Here's how the part is built. I have some questions about the finished solid (model axes, mm). A direction names the side the tool comes from. Give positions to 0.01 mm unless a question says otherwise; leave off trailing zeros. Order: outer loops, then holes, each group sorted by start corner. A loop starts at its lowest first (then second) coordinate and runs counter-clockwise, first axis right, second up.
from build123d import *

# Parameters (mm, degrees)
SKETCH1_R           = 3
SKETCH1_R_2         = 1.2
SKETCH1_R_3         = 6.35
SKETCH1_W           = 5
SKETCH1_H           = 15
SKETCH1_W_2         = 10
SKETCH1_H_2         = 17.5
BOSS_EXTRUDE1_DEPTH = 5
SKETCH2_W           = 38
SKETCH2_H           = 55
BOSS_EXTRUDE2_DEPTH = 5
FILLET1_R           = 5


with BuildPart() as part:
    # Sketch1 → Boss-Extrude1 (new body)
    with BuildSketch(Plane.XY):
        Polygon((-23.5, 65), (23.5, 65), (23.5, 0), (0, 0), (-23.5, 0), align=None)
        with Locations((16, 51)):
            Circle(SKETCH1_R, mode=Mode.SUBTRACT)
        with Locations((16, 19.2)):
            Circle(SKETCH1_R_2, mode=Mode.SUBTRACT)
        with Locations((16, 59)):
            Circle(SKETCH1_R_2, mode=Mode.SUBTRACT)
        with Locations(Location((-16, 59, 0), (0, 0, 180))):
            Circle(SKETCH1_R_2, mode=Mode.SUBTRACT)
        with Locations(Location((-16, 19.2, 0), (0, 0, 180))):
            Circle(SKETCH1_R_2, mode=Mode.SUBTRACT)
        with Locations(Location((-16, 51, 0), (0, 0, 180))):
            Circle(SKETCH1_R, mode=Mode.SUBTRACT)
        with Locations((0, 15)):
            Circle(SKETCH1_R_3, mode=Mode.SUBTRACT)
        with Locations((16, 33.5)):
            Rectangle(SKETCH1_W, SKETCH1_H, mode=Mode.SUBTRACT)
        with Locations((-2.5, 45.25)):
            Rectangle(SKETCH1_W_2, SKETCH1_H_2, mode=Mode.SUBTRACT)
        with Locations((-16, 33.5)):
            Rectangle(SKETCH1_W, SKETCH1_H, mode=Mode.SUBTRACT)
    extrude(amount=BOSS_EXTRUDE1_DEPTH)

    # Sketch2 → Boss-Extrude2 (add)
    with BuildSketch(Plane(origin=(0, 0, 0), x_dir=(-1, 0, 0), z_dir=(0, 0, -1))):
        with Locations((-42.5, 37.5)):
            Rectangle(SKETCH2_W, SKETCH2_H)
        with BuildLine():
            Line((-37.5, 44.5), (-37.5, 29.5))
            ThreePointArc((-37.5, 29.5), (-40.5, 26.5), (-43.5, 29.5))
            Line((-43.5, 29.5), (-43.5, 44.5))
            ThreePointArc((-43.5, 44.5), (-40.5, 47.5), (-37.5, 44.5))
        make_face(mode=Mode.SUBTRACT)
        with BuildLine():
            Line((-23.7, 60), (-23.7, 47.5))
            ThreePointArc((-23.7, 47.5), (-25, 46.2), (-26.3, 47.5))
            Line((-26.3, 47.5), (-26.3, 60))
            ThreePointArc((-26.3, 60), (-25, 61.3), (-23.7, 60))
        make_face(mode=Mode.SUBTRACT)
        with BuildLine():
            Line((-54.668271165, 60), (-54.668271165, 47.5))
            ThreePointArc((-54.668271165, 47.5), (-55.968271165, 46.2), (-57.268271165, 47.5))
            Line((-57.268271165, 47.5), (-57.268271165, 60))
            ThreePointArc((-57.268271165, 60), (-55.968271165, 61.3), (-54.668271165, 60))
        make_face(mode=Mode.SUBTRACT)
        with BuildLine():
            Line((-23.7, 29), (-23.7, 16.5))
            ThreePointArc((-23.7, 16.5), (-25, 15.2), (-26.3, 16.5))
            Line((-26.3, 16.5), (-26.3, 29))
            ThreePointArc((-26.3, 29), (-25, 30.3), (-23.7, 29))
        make_face(mode=Mode.SUBTRACT)
        with BuildLine():
            Line((-54.668271165, 29), (-54.668271165, 16.5))
            ThreePointArc((-54.668271165, 16.5), (-55.968271165, 15.2), (-57.268271165, 16.5))
            Line((-57.268271165, 16.5), (-57.268271165, 29))
            ThreePointArc((-57.268271165, 29), (-55.968271165, 30.3), (-54.668271165, 29))
        make_face(mode=Mode.SUBTRACT)
    extrude(amount=-BOSS_EXTRUDE2_DEPTH)

    # Fillet1
    fillet1_edges = [part.edges().sort_by_distance(p)[0] for p in [
        (23.5, 0, 2.5),
        (-23.5, 0, 2.5),
        (-23.5, 65, 2.5),
        (23.5, 10, 2.5),
        (61.5, 10, 2.5),
        (61.5, 65, 2.5),
    ]]
    fillet(fillet1_edges, radius=FILLET1_R - 0.0001)  # a hair under: the kernel refuses the full size


solid = part.part
Q1. If we section it at D-D on y = 33: List the corners of the cut face in (x, z) for me.
Filled sheet:
outline: (-23.5, 0) - (-18.5, 0) - (-18.5, 5) - (-23.5, 5) - close; (-13.5, 0) - (13.5, 0) - (13.5, 5) - (-13.5, 5) - close; (18.5, 0) - (37.5, 0) - (37.5, 5) - (18.5, 5) - close; (43.5, 0) - (61.5, 0) - (61.5, 5) - (43.5, 5) - close
Q2. I'm going to push flat-ended pins straight in: P1, Ø1.5, axis at x = 48.5, z = 3.5, coming from the -Y side; P2, Ø1.9, axis at x = 16, y = 19.2, coming from the +Z side (3 decimals). Where does each tip first touch, or does it pass through?
Filled sheet:
P1: stops at y = 10
P2: passes through
Q3. Thinking about a two-plate mould opening in X: for faces 1 (the face through (24.93, 8.5, 2.54)), 2 (the face through (-16, 26, 2)), 3 (the face through (0, 0, 2)), which applies, released by +X, released by -X, zero draft, split by the parting line, or undercut?
Filled sheet:
face 1: released by +X
face 2: undercut
face 3: zero draft
Q4. If we section it at C-C on x = 40.5: List the corners of the cut face in (y, z) for me, plus the area to 3 significant figures.
Filled sheet:
outline: (10, 0) - (26.5, 0) - (26.5, 5) - (10, 5) - close; (47.5, 0) - (65, 0) - (65, 5) - (47.5, 5) - close
area: 170 mm2
Q5. If we section it at A-A on x = -16: List the corners of the cut face in (y, z) for me, plus the area to 3 significant figures.
Filled sheet:
outline: (0, 0) - (18, 0) - (18, 5) - (0, 5) - close; (20.4, 0) - (26, 0) - (26, 5) - (20.4, 5) - close; (41, 0) - (48, 0) - (48, 5) - (41, 5) - close; (54, 0) - (57.8, 0) - (57.8, 5) - (54, 5) - close; (60.2, 0) - (65, 0) - (65, 5) - (60.2, 5) - close
area: 196 mm2
Q6. I need wall thicknesses on L1, parallel to X at y = 39.5, z = 2.1; L2, parallel to X at y = 31, z = 0.7; L3, parallel to Y at x = 16, z = 1.7. Which ranges of each line are inside material? Lowest first, please.
Filled sheet:
L1: x = -23.5 to -18.5, -13.5 to -7.5, 2.5 to 13.5, 18.5 to 37.5, 43.5 to 61.5
L2: x = -23.5 to -18.5, -13.5 to 13.5, 18.5 to 37.5, 43.5 to 61.5
L3: y = 0 to 18, 20.4 to 26, 41 to 48, 54 to 57.8, 60.2 to 65
Q7. For faces 4 (the face through (61.5, 37, 2)), 5 (the face through (43, 10, 2)), 6 (the face through (25, 61.3, 2.5)), which set-ups out of +Z, -Z, +X, -X, +Y, -Y let a thin tool reach every point of the face, with its end or its side?
Filled sheet:
face 4: +Z, -Z, +X, +Y, -Y
face 5: +Z, -Z, +X, -Y
face 6: +Z, -Z
Q8. If we section it at B-B on y = 51: List the corners of the cut face in (x, z) for me.
Filled sheet:
outline: (-23.5, 0) - (-19, 0) - (-19, 5) - (-23.5, 5) - close; (-13, 0) - (-7.5, 0) - (-7.5, 5) - (-13, 5) - close; (2.5, 0) - (13, 0) - (13, 5) - (2.5, 5) - close; (19, 0) - (23.7, 0) - (23.7, 5) - (19, 5) - close; (26.3, 0) - (54.67, 0) - (54.67, 5) - (26.3, 5) - close; (57.27, 0) - (61.5, 0) - (61.5, 5) - (57.27, 5) - close
